CAD build for the part. Positions are in the model's coordinates, mm. A direction names the side the tool comes from. Give positions to 0.01 mm unless a question says otherwise; leave off trailing zeros. Write each loop counter-clockwise with the first axis right and the second up, starting at its lowest first coordinate (ties: lowest second). Pieces come first, ordered by that corner, then holes. Notation, with made-up numbers: (-31.75, -37) - (-3.75, -37) arc R36 cw to (-3.75, 0) - close; hole circle Ø2 at (-4, 9.5). An arc over 180 degrees is marked (long way). Answer as a JSON object with one key per item and string values.
from build123d import *

# Parameters (mm, degrees)
F0_R     = 2.25
F0_R_2   = 2.5
F1_DEPTH = 6.5
F2_SIZE  = 1.5
F3_W     = 5
F3_H     = 8
F3_H_2   = 7
F4_DEPTH = 3.5


with BuildPart() as f1:
    # F0 (on Top) → F1 (new body)
    with BuildSketch(Plane.XY):
        Polygon((-21.849313, 8.429525), (-36.849313, 8.429525), (-36.849313, -81.570475), (33.150687, -81.570475), (33.150687, -66.570475), (23.150687, -66.570475), (-21.849313, -66.570475), align=None)
        with Locations((-29.349313, -74.020133)):
            Circle(F0_R, mode=Mode.SUBTRACT)
        with Locations((12.650687, -73.985228)):
            Circle(F0_R, mode=Mode.SUBTRACT)
        with Locations((23.150687, -73.976502)):
            Circle(F0_R_2, mode=Mode.SUBTRACT)
        with Locations((-29.349313, -22.020115)):
            Circle(F0_R, mode=Mode.SUBTRACT)
        with Locations((-29.349313, -0.070475)):
            Circle(F0_R_2, mode=Mode.SUBTRACT)
    extrude(amount=F1_DEPTH)

    # F2
    f2_edges = [f1.edges().sort_by_distance(p)[0] for p in [
        (-21.849313, 8.429525, 3.25),
        (-36.849313, 8.429525, 3.25),
        (-36.849313, -81.570475, 3.25),
        (-21.849313, -66.570475, 3.25),
        (33.150687, -66.570475, 3.25),
        (33.150687, -81.570475, 3.25),
    ]]
    chamfer(f2_edges, length=F2_SIZE)

    # F3 (on face) → F4 (cut)
    with BuildSketch(Plane.XY.offset(6.5)):
        with Locations((-27.349313, -42.020133)):
            Rectangle(F3_W, F3_H)
        with Locations((-25.349313, -57.520133)):
            Rectangle(F3_W, F3_H_2)
    extrude(amount=-F4_DEPTH, mode=Mode.SUBTRACT)


solid = f1.part
Item 1: Which spindle directions (+Z, -Z, +X, -X, +Y, -Y) get a long thin tool onto all of the face, cutting with end or side? Do faces 4 (the cylindrical face through (-31.847, 0.039, 3.204)), 5 (the flat face through (-27, -46.02, 5)), 6 (the flat face through (-21.849, -30, 3)). Say none if no direction does.
Entries:
{"face 4": "+Z, -Z", "face 5": "+Z", "face 6": "+Z, -Z, +X, +Y"}
Item 2: Cut at D-D (y = -53). Give the cut face in (x, z), and give its area (3 significant figures).
Entries:
{"outline": "(-36.85, 0) - (-21.85, 0) - (-21.85, 6.5) - (-36.85, 6.5) - close", "area": "97.5 mm2"}
Item 3: Probe line 1 (Y direction, x = -25.5, z = 5.25); line 2 (X direction, y = -41, z = 4.5); line 3 (X direction, y = 0, z = 4). List the from-to ranges inside material, lowest first. Write a range as from..to.
Entries:
{"line 1": "-81.57..-61.02, -54.02..-46.02, -38.02..8.43", "line 2": "-36.85..-29.85, -24.85..-21.85", "line 3": "-36.85..-31.85, -26.85..-21.85"}
Item 4: Flat gauge pins, fed straight in: P1, Ø2.5, axis at x = -26, y = -58.5, coming from the +Z side; P2, Ø4.5, axis at x = -29.35, y = -0.07, coming from the +Z side; P3, Ø3, axis at y = -27.5, z = 3.5, coming from the +X side. Where does each tip first touch, or does it go through?
Entries:
{"P1": "z = 3", "P2": "through", "P3": "x = -21.85"}
Item 5: Cut at A-A (y = -1.5). Give the cut face in (x, z).
Entries:
{"outline": "(-36.85, 0) - (-31.4, 0) - (-31.4, 6.5) - (-36.85, 6.5) - close; (-27.3, 0) - (-21.85, 0) - (-21.85, 6.5) - (-27.3, 6.5) - close"}
Item 6: Mould opens along Y. For faces 1 (the flat face through (-23, -46, 0)), 2 (the flat face through (-29, 8.43, 3)), 3 (the flat face through (-25, -57, 3)) say: +Y half, -Y half, draft (parallel to the pull), parting line (faces both ways), or undercut.
Entries:
{"face 1": "draft", "face 2": "+Y half", "face 3": "undercut"}
Item 7: Cut at B-B (x = 24.5). Give the cut face in (y, z), and give its area (3 significant figures).
Entries:
{"outline": "(-81.57, 0) - (-76.08, 0) - (-76.08, 6.5) - (-81.57, 6.5) - close; (-71.87, 0) - (-66.57, 0) - (-66.57, 6.5) - (-71.87, 6.5) - close", "area": "70.1 mm2"}
Item 8: Cut at C-C (z = 4.5). Give the cut face in (x, y).
Entries:
{"outline": "(-36.85, -80.07) - (-35.35, -81.57) - (31.65, -81.57) - (33.15, -80.07) - (33.15, -68.07) - (31.65, -66.57) - (-20.35, -66.57) - (-21.85, -65.07) - (-21.85, 6.93) - (-23.35, 8.43) - (-35.35, 8.43) - (-36.85, 6.93) - close; hole circle Ø5 at (-29.35, -0.07); hole circle Ø4.5 at (-29.35, -74.02); hole circle Ø4.5 at (-29.35, -22.02); hole (-29.85, -46.02) - (-24.85, -46.02) - (-24.85, -38.02) - (-29.85, -38.02) - close; hole (-27.85, -61.02) - (-22.85, -61.02) - (-22.85, -54.02) - (-27.85, -54.02) - close; hole circle Ø4.5 at (12.65, -73.99); hole circle Ø5 at (23.15, -73.98)"}
